Geometry check sheet. Reference: the model listing, model coordinates, mm. Face numbers are marked on the shaded views. A direction names the side the tool comes from. Round coordinates to 2 decimals unless told otherwise and drop trailing zeros. Write each loop counter-clockwise with the first axis right and the second up, starting at its lowest first coordinate (ties: lowest second). Pieces come first, ordered by that corner, then holes. Notation, with made-up numbers: (-5.75, 0) - (21.25, 0) arc R8 cw to (21.25, 11) - close; hole circle Ø6 at (33.25, -12.5). An arc over 180 degrees is marked (long way). One line per question, with ' | ' between items. Start each with the question number.
from build123d import *

# Parameters (mm, degrees)
SKETCH1_W           = 56
SKETCH1_H           = 100
BOSS_EXTRUDE1_DEPTH = 50
CUT_EXTRUDE2_DEPTH  = 116.256236274
SKETCH7_R           = 22.5
SKETCH7_R_2         = 10
CUT_EXTRUDE4_DEPTH  = 9
CUT_EXTRUDE5_DEPTH  = 35.5
CUT_EXTRUDE6_DEPTH  = 3
CUT_EXTRUDE7_DEPTH  = 9
SKETCH12_W          = 16
SKETCH12_H          = 17.5
CUT_EXTRUDE8_DEPTH  = 77.052613367


with BuildPart() as part:
    # Sketch1 → Boss-Extrude1 (new body)
    with BuildSketch(Plane(origin=(0, 0, 0), x_dir=(1, 0, 0), z_dir=(0, 1, 0))):
        Rectangle(SKETCH1_W, SKETCH1_H)
    extrude(amount=BOSS_EXTRUDE1_DEPTH)

    # Sketch3 → Cut-Extrude2 (cut, through all)
    with BuildSketch(Plane.XY.offset(50)):
        Polygon((-0.5, 10), (-2, 50), (2, 50), (0.5, 10), align=None)
    extrude(amount=-CUT_EXTRUDE2_DEPTH, mode=Mode.SUBTRACT)

    # Sketch7 → Cut-Extrude4 (cut)
    with BuildSketch(Plane(origin=(0, 50, 0), x_dir=(1, 0, 0), z_dir=(0, 1, 0))):
        with Locations((22, 0)):
            Circle(SKETCH7_R)
        with Locations((22, 0)):
            Circle(SKETCH7_R_2, mode=Mode.SUBTRACT)
    cut_extrude4 = extrude(amount=-CUT_EXTRUDE4_DEPTH, mode=Mode.SUBTRACT)

    # Sketch9 → Cut-Extrude5 (cut)
    with BuildSketch(Plane(origin=(0, 50, 0), x_dir=(1, 0, 0), z_dir=(0, 1, 0))):
        with BuildLine():
            Line((14.5, 6.614378278), (14.5, -6.614378278))
            ThreePointArc((14.5, -6.614378278), (32, 0), (14.5, 6.614378278))
        make_face()
    cut_extrude5 = extrude(amount=-CUT_EXTRUDE5_DEPTH, mode=Mode.SUBTRACT)

    # Sketch10 → Cut-Extrude6 (cut)
    with BuildSketch(Plane(origin=(0, 14.5, 0), x_dir=(1, 0, 0), z_dir=(0, 1, 0))):
        with BuildLine():
            Line((18, 3), (18, -3))
            ThreePointArc((18, -3), (27, 0), (18, 3))
        make_face()
    cut_extrude6 = extrude(amount=-CUT_EXTRUDE6_DEPTH, mode=Mode.SUBTRACT)

    # Sketch11 → Cut-Extrude7 (cut)
    with BuildSketch(Plane(origin=(0, 50, 0), x_dir=(1, 0, 0), z_dir=(0, 1, 0))):
        with BuildLine():
            Line((14.5, 6.614378278), (14.5, -6.614378278))
            ThreePointArc((14.5, -6.614378278), (12, 0), (14.5, 6.614378278))
        make_face()
    cut_extrude7 = extrude(amount=-CUT_EXTRUDE7_DEPTH, mode=Mode.SUBTRACT)

    # Mirror1: Cut-Extrude4, Cut-Extrude5, Cut-Extrude6, Cut-Extrude7 across plane
    add(cut_extrude4.mirror(Plane(origin=(0, 0, 0), x_dir=(0, 0, 1), z_dir=(1, 0, 0))), mode=Mode.SUBTRACT)
    add(cut_extrude5.mirror(Plane(origin=(0, 0, 0), x_dir=(0, 0, 1), z_dir=(1, 0, 0))), mode=Mode.SUBTRACT)
    add(cut_extrude6.mirror(Plane(origin=(0, 0, 0), x_dir=(0, 0, 1), z_dir=(1, 0, 0))), mode=Mode.SUBTRACT)
    add(cut_extrude7.mirror(Plane(origin=(0, 0, 0), x_dir=(0, 0, 1), z_dir=(1, 0, 0))), mode=Mode.SUBTRACT)

    # Sketch12 → Cut-Extrude8 (cut, through all)
    with BuildSketch(Plane(origin=(0, 50, 0), x_dir=(1, 0, 0), z_dir=(0, 1, 0))):
        with Locations((-20, 41.25)):
            Rectangle(SKETCH12_W, SKETCH12_H)
        with Locations((20, 41.25)):
            Rectangle(SKETCH12_W, SKETCH12_H)
        with Locations((-20, -41.25)):
            Rectangle(SKETCH12_W, SKETCH12_H)
        with Locations((20, -41.25)):
            Rectangle(SKETCH12_W, SKETCH12_H)
    extrude(amount=-CUT_EXTRUDE8_DEPTH, mode=Mode.SUBTRACT)


solid = part.part
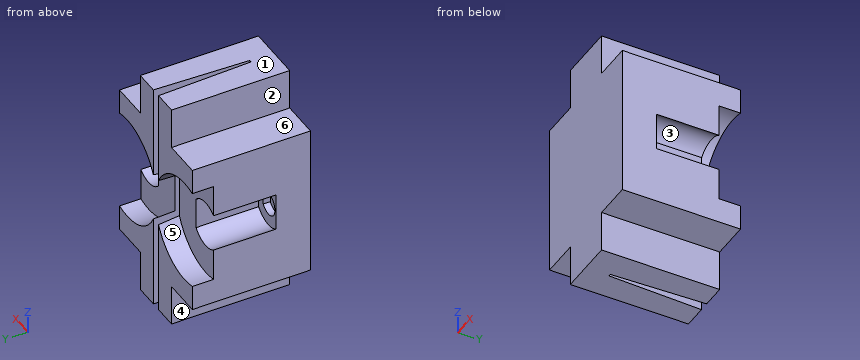
Q1. Section check C-C, the plane y = 46.5. Record the cut outline in (x, z), then the cut area to 3 significant figures.
Q2. Section check D-D, the plane x = -22. Record the cut outline in (y, z).
Q3. Go/stop test with flat-tipped pins: P1, Ø4, axis at y = 25, z = 2.5, coming from the +X side; P2, Ø6.5, axis at y = 26.5, z = 1, coming from the -X side; P3, Ø13, axis at x = -23.5, y = 32, coming from the +Z side. Record where each tip stops, or that it passes through.
Q4. Draft check along X on the marked faces 1, 2 and 3. Enter one of: pulls with the +X half, pulls with the -X half, needs draft (parallel to the pull), parting line crosses it, or undercut.
Q5. Section check A-A, the plane y = 22. Record the cut outline in (x, z), then the cut area to 3 significant figures.
Q6. Set-up check for the marked faces 4, 5 and 6: record each of +Z, -Z, +X, -X, +Y, -Y from which the full face is reachable in a straight line by a thin tool's end or side.
Q7. Section check B-B, the plane z = 0. Record the cut outline in (x, y).
Q8. Thickness scan on line 1 (Z direction, x = 22, y = 12.85); line 2 (Z direction, x = -17.5, y = 4.5); line 3 (X direction, y = 12.85, z = 0). Record the ranges inside material, lowest first.
Result sheet:
1) outline: (-28, -32.5) - (-12, -32.5) - (-12, -50) - (-1.87, -50) - (-1.87, -10.05) arc R22.5 cw to (-28, -21.69) - close; (-28, 21.69) arc R22.5 cw to (-1.87, 10.05) - (-1.87, 50) - (-12, 50) - (-12, 32.5) - (-28, 32.5) - close; (1.87, -50) - (12, -50) - (12, -32.5) - (28, -32.5) - (28, -21.69) arc R22.5 cw to (1.87, -10.05) - close; (1.87, 10.05) arc R22.5 cw to (28, 21.69) - (28, 32.5) - (12, 32.5) - (12, 50) - (1.87, 50) - close | area: 2,050 mm²
2) outline: (0, -32.5) - (50, -32.5) - (50, -22.5) - (41, -22.5) - (41, -10) - (14.5, -10) - (14.5, -5) - (11.5, -5) - (11.5, 5) - (14.5, 5) - (14.5, 10) - (41, 10) - (41, 22.5) - (50, 22.5) - (50, 32.5) - (0, 32.5) - close
3) P1: x = 14.5 | P2: x = -14.5 | P3: z = 32.5
4) face 1: needs draft | face 2: pulls with the -X half | face 3: undercut
5) outline: (-28, -32.5) - (-12, -32.5) - (-12, -50) - (-0.95, -50) - (-0.95, 50) - (-12, 50) - (-12, 32.5) - (-28, 32.5) - (-28, 8) arc R10 cw to (-14.5, 6.61) - (-14.5, -6.61) arc R10 cw to (-28, -8) - close; (0.95, -50) - (12, -50) - (12, -32.5) - (28, -32.5) - (28, -8) arc R10 cw to (14.5, -6.61) - (14.5, 6.61) arc R10 cw to (28, 8) - (28, 32.5) - (12, 32.5) - (12, 50) - (0.95, 50) - close | area: 3,800 mm²
6) face 4: -Z, -X, +Y, -Y | face 5: +Y | face 6: +Z, -X, +Y, -Y
7) outline: (-28, 0) - (28, 0) - (28, 14.5) - (27, 14.5) - (27, 11.5) - (18, 11.5) - (18, 14.5) - (14.5, 14.5) - (14.5, 41) - (1.66, 41) - (0.5, 10) - (-0.5, 10) - (-1.66, 41) - (-14.5, 41) - (-14.5, 14.5) - (-18, 14.5) - (-18, 11.5) - (-27, 11.5) - (-27, 14.5) - (-28, 14.5) - close
8) line 1: -32.5 to -5, 5 to 32.5 | line 2: -32.5 to 32.5 | line 3: -28 to -27, -18 to -0.61, 0.61 to 18, 27 to 28
